from build123d import *

# Parameters (mm, degrees)
SKETCH1_R               = 29.21
BOSS_EXTRUDE1_DEPTH     = 33.02
SKETCH2_W               = 60.96
SKETCH2_H               = 58.42
BOSS_EXTRUDE2_DEPTH     = 40.64
SKETCH3_R               = 12.7
CUT_EXTRUDE1_DEPTH      = 59.42
SKETCH4_R               = 25.4
CUT_EXTRUDE2_DEPTH      = 33.02
CUT_EXTRUDE3_DEPTH      = 1
CUT_EXTRUDE3_DEPTH_BACK = 59.42


with BuildPart() as part:
    # Sketch1 → Boss-Extrude1 (new body)
    with BuildSketch(Plane(origin=(0, 0, 0), x_dir=(1, 0, 0), z_dir=(0, 1, 0))):
        Circle(SKETCH1_R)
    extrude(amount=BOSS_EXTRUDE1_DEPTH)

    # Sketch2 → Boss-Extrude2 (add)
    with BuildSketch(Plane.XZ):
        Rectangle(SKETCH2_W, SKETCH2_H)
    extrude(amount=BOSS_EXTRUDE2_DEPTH)

    # Sketch3 → Cut-Extrude1 (cut, through all)
    with BuildSketch(Plane.XY.offset(29.21)):
        with Locations((0, -22.86)):
            Circle(SKETCH3_R)
    extrude(amount=-CUT_EXTRUDE1_DEPTH, mode=Mode.SUBTRACT)

    # Sketch4 → Cut-Extrude2 (cut)
    with BuildSketch(Plane(origin=(0, 33.02, 0), x_dir=(1, 0, 0), z_dir=(0, 1, 0))):
        Circle(SKETCH4_R)
    extrude(amount=-CUT_EXTRUDE2_DEPTH, mode=Mode.SUBTRACT)

    # Sketch5 → Cut-Extrude3 (cut, two sides)
    with BuildSketch(Plane.XY.offset(29.21)) as cut_extrude3_sk:
        with BuildLine():
            Line((30.48, -14.429530232), (13.554352704, -34.366864159))
            ThreePointArc((13.554352704, -34.366864159), (7.467809426, -38.995681652), (0, -40.64))
            Line((0, -40.64), (30.48, -40.64))
            Line((30.48, -40.64), (30.48, -14.429530232))
        make_face()
        with BuildLine():
            Line((-30.48, -40.64), (0, -40.64))
            ThreePointArc((0, -40.64), (-7.467809426, -38.995681652), (-13.554352704, -34.366864159))
            Line((-13.554352704, -34.366864159), (-30.48, -14.429530232))
            Line((-30.48, -14.429530232), (-30.48, -40.64))
        make_face()
    extrude(amount=CUT_EXTRUDE3_DEPTH, mode=Mode.SUBTRACT)
    extrude(cut_extrude3_sk.sketch, amount=-CUT_EXTRUDE3_DEPTH_BACK, mode=Mode.SUBTRACT)


solid = part.part
CAD build for the part. Positions are in the model's coordinates, mm. A direction names the side the tool comes from. Coordinates: 2 decimals unless noted, no trailing zeros. Order: outer loops, then holes, each group sorted by start corner. A loop starts at its lowest first (then second) coordinate and runs counter-clockwise, first axis right, second up.
Item 1: Pin check, flat tips, straight feed: pin 1 Ø24.5 at (x, z) = (-12.5, 14) entering from +Y; pin 2 Ø10 at (y, z) = (20, 3) entering from -X; pin 3 Ø6 at (x, z) = (19.5, -9) entering from +Y; pin 4 Ø6 at (x, z) = (-11.5, 3) entering from -Y. Stop position of each tip, or through.
Check sheet entries:
pin 1: stops at y = 33.02
pin 2: stops at x = -29.21
pin 3: stops at y = 0
pin 4: stops at y = -38.48
Item 2: Band-saw the part on A-A on y = -22.86. List the corners of the cut face in (x, z), plus the area to 3 significant figures.
Check sheet entries:
outline: (-23.32, -29.21) - (-12.7, -29.21) - (-12.7, 29.21) - (-23.32, 29.21) - close; (12.7, -29.21) - (23.32, -29.21) - (23.32, 29.21) - (12.7, 29.21) - close
area: 1,240 mm2
Item 3: 3-axis set-ups, long thin cutter, end or side, ignore diameter. For faces 1 (the face through (-29, 0, 7)), 2 (the face through (30, 0, 2)), 3 (the face through (-5.506, 16.741, 24.796)), 4 (the face through (-1.653, -10.268, 0.409)): which of +Z, -Z, +X, -X, +Y, -Y reach the whole face in a straight line?
Check sheet entries:
face 1: -X, +Y
face 2: +X, +Y
face 3: +Y
face 4: +Z, -Z
Item 4: Band-saw the part on D-D on y = 28.5. List the corners of the cut face in (x, z).
Check sheet entries:
outline: circle Ø58.42 at (0, 0); hole circle Ø50.8 at (0, 0)
Item 5: Two-plate mould, pull along Z, no slides. Class faces 5 (the face through (0, 0, 0)), 6 (the face through (-7, -11, -29.21)), 7 (the face through (-21.53, 16.28, -19.74)), 8 (the face through (-30.48, -7, 0)): +Z half, -Z half, draft (parallel to the pull), parting line (faces both ways), or undercut.
Check sheet entries:
face 5: undercut
face 6: -Z half
face 7: parting line
face 8: draft
Item 6: Drill centre lines: L1, parallel to X at y = 8, z = 0; L2, parallel to Y at x = 0, z = 14. Where is each one in solid material? Low to high.
Check sheet entries:
L1: x = -29.21 to -25.4, 25.4 to 29.21
L2: y = -40.64 to -35.56, -10.16 to 0
Item 7: Band-saw the part on C-C on x = 10.5. List the corners of the cut face in (y, z), plus the area to 3 significant figures.
Check sheet entries:
outline: (-37.21, -29.21) - (-30, -29.21) - (-30, 29.21) - (-37.21, 29.21) - close; (-15.72, -29.21) - (0, -29.21) - (0, -27.26) - (33.02, -27.26) - (33.02, -23.13) - (0, -23.13) - (0, 23.13) - (33.02, 23.13) - (33.02, 27.26) - (0, 27.26) - (0, 29.21) - (-15.72, 29.21) - close
area: 1,610 mm2
Item 8: Band-saw the part on B-B on z = -7. List the corners of the cut face in (x, y), plus the area to 3 significant figures.
Check sheet entries:
outline: (-30.48, -14.43) - (-13.55, -34.37) arc R17.78 ccw to (13.55, -34.37) - (30.48, -14.43) - (30.48, 0) - (28.36, 0) - (28.36, 33.02) - (24.42, 33.02) - (24.42, 0) - (-24.42, 0) - (-24.42, 33.02) - (-28.36, 33.02) - (-28.36, 0) - (-30.48, 0) - close; hole circle Ø25.4 at (0, -22.86)
area: 1,630 mm2
